```python
from build123d import *

# Parameters (mm, degrees)
F0_W      = 28
F0_H      = 26
F0_R      = 1.55
F1_DEPTH  = 6
F5_DEPTH  = 6.5
F6_DEPTH  = 10
F9_R      = 1.6
F10_DEPTH = 4
F11_DEPTH = 25
F12_START = -6
F9_R_2    = 3.5
F12_DEPTH = 19
F13_R     = 1.6
F14_DEPTH = 4
F15_DEPTH = 25
F16_START = -6
F13_R_2   = 3.5
F16_DEPTH = 19
F17_R     = 3.5
F18_DEPTH = 2
F19_DEPTH = 25


# Not quite as in the source:
# - a fillet or chamfer that OpenCascade refuses, or shapes differently, is made with other operations: its cross-section is extruded or revolved along the edge and cut away or added


with BuildPart() as f1:
    # F0 (on Top) → F1 (new body)
    with BuildSketch(Plane.XY):
        Rectangle(F0_W, F0_H)
        with Locations((0, -7)):
            Circle(F0_R, mode=Mode.SUBTRACT)
        with Locations((-9, 8)):
            Circle(F0_R, mode=Mode.SUBTRACT)
        with Locations((9, 8)):
            Circle(F0_R, mode=Mode.SUBTRACT)
    extrude(amount=F1_DEPTH)

    # F4 (on face) → F5 (join)
    with BuildSketch(Plane(origin=(3.5, 0, -6.0621778265), x_dir=(0.8660254038, 0, 0.5), z_dir=(-0.5, 0, 0.8660254038))):
        with BuildLine():
            Line((12.124355653, -13), (27.124355653, -13))
            ThreePointArc((27.124355653, -13), (14.124355653, 0), (27.124355653, 13))
            Line((27.124355653, 13), (12.124355653, 13))
            Line((12.124355653, 13), (12.124355653, -13))
        make_face()
        with BuildLine():
            ThreePointArc((27.124355653, 13), (14.124355653, 0), (27.124355653, -13))
            ThreePointArc((27.124355653, -13), (36.3167438084, -9.1923881554), (40.124355653, 0))
            ThreePointArc((40.124355653, 0), (36.3167438084, 9.1923881554), (27.124355653, 13))
        make_face()
    extrude(amount=F5_DEPTH)

    # F4 (on face) → F6 (join)
    with BuildSketch(Plane(origin=(3.5, 0, -6.0621778265), x_dir=(0.8660254038, 0, 0.5), z_dir=(-0.5, 0, 0.8660254038))):
        with BuildLine():
            ThreePointArc((27.124355653, 13), (14.124355653, 0), (27.124355653, -13))
            ThreePointArc((27.124355653, -13), (36.3167438084, -9.1923881554), (40.124355653, 0))
            ThreePointArc((40.124355653, 0), (36.3167438084, 9.1923881554), (27.124355653, 13))
        make_face()
    extrude(amount=F6_DEPTH)

    # F7: chamfer of 2 on 1 edges, made by hand

    # F7_s1 → F7_t2 (revolve, cut)
    with BuildSketch(Plane.XZ):
        with BuildLine():
            Line((34.3259853721, 20.9074977067), (31.4393864323, 21.6809595615))
            Line((31.4393864323, 21.6809595615), (31.4193864323, 21.7156005776))
            ThreePointArc((31.4193864323, 21.7156005776), (32.3381910048, 22.1807529184), (33.228711306, 22.694895054))
            Line((33.228711306, 22.694895054), (33.2833523221, 22.6802540378))
            ThreePointArc((33.2833523221, 22.6802540378), (33.7974944577, 21.7897337366), (34.3606263882, 20.9274977067))
            Line((34.3606263882, 20.9274977067), (34.3259853721, 20.9074977067))
        make_face()
    revolve(axis=Axis((21.9903810568, 0, 16.1602540378), (0.5, 0, -0.8660254038)), mode=Mode.SUBTRACT)

    # F8: F1 across plane


with BuildPart() as f1_1:
    add(f1.part)
    add(f1.part.mirror(Plane.YZ))

    # F9 (on face) → F10 (cut)
    with BuildSketch(Plane(origin=(-1.5, 0, 2.5980762114), x_dir=(0.8660254038, 0, 0.5), z_dir=(-0.5, 0, 0.8660254038))):
        with BuildLine():
            ThreePointArc((23.9821806278, -10.5416666667), (27.124355653, -11.0000000001), (30.2665306781, -10.5416666667))
            ThreePointArc((30.2665306781, -10.5416666667), (30.5337260192, -9.7913240209), (30.624355653, -9))
            ThreePointArc((30.624355653, -9), (26.3330316321, -5.5906296338), (23.9821806278, -10.5416666667))
        make_face()
        with Locations((27.124355653, -9)):
            Circle(F9_R, mode=Mode.SUBTRACT)
        with BuildLine():
            ThreePointArc((23.9821806278, -10.5416666667), (27.124355653, -12.5), (30.2665306781, -10.5416666667))
            ThreePointArc((30.2665306781, -10.5416666667), (27.124355653, -11.0000000001), (23.9821806278, -10.5416666667))
        make_face()
        with BuildLine():
            ThreePointArc((22.624355653, 0), (20.2336206122, 3.3195679312), (16.3274806529, 2.1041602206))
            ThreePointArc((16.3274806529, 2.1041602206), (16.1243556529, 0), (16.3274806529, -2.1041602206))
            ThreePointArc((16.3274806529, -2.1041602206), (20.2336206122, -3.3195679312), (22.624355653, 0))
        make_face()
        with Locations((19.124355653, 0)):
            Circle(F9_R, mode=Mode.SUBTRACT)
        with BuildLine():
            ThreePointArc((16.3274806529, -2.1041602206), (16.1243556529, 0), (16.3274806529, 2.1041602206))
            ThreePointArc((16.3274806529, 2.1041602206), (15.624355653, 0), (16.3274806529, -2.1041602206))
        make_face()
        with BuildLine():
            ThreePointArc((30.624355653, 9), (30.5337260192, 9.7913240209), (30.2665306781, 10.5416666667))
            ThreePointArc((30.2665306781, 10.5416666667), (27.124355653, 11.0000000001), (23.9821806278, 10.5416666667))
            ThreePointArc((23.9821806278, 10.5416666667), (26.3330316321, 5.5906296338), (30.624355653, 9))
        make_face()
        with Locations((27.124355653, 9)):
            Circle(F9_R, mode=Mode.SUBTRACT)
        with BuildLine():
            ThreePointArc((23.9821806278, 10.5416666667), (27.124355653, 11.0000000001), (30.2665306781, 10.5416666667))
            ThreePointArc((30.2665306781, 10.5416666667), (27.124355653, 12.5), (23.9821806278, 10.5416666667))
        make_face()
        with BuildLine():
            ThreePointArc((38.124355653, 0), (38.0734566435, 1.0569709078), (37.9212306531, 2.1041602206))
            ThreePointArc((37.9212306531, 2.1041602206), (31.624355653, 0), (37.9212306531, -2.1041602206))
            ThreePointArc((37.9212306531, -2.1041602206), (38.0734566435, -1.0569709078), (38.124355653, 0))
        make_face()
        with Locations((35.124355653, 0)):
            Circle(F9_R, mode=Mode.SUBTRACT)
        with BuildLine():
            ThreePointArc((37.9212306531, -2.1041602206), (38.4439235842, -1.1092649593), (38.624355653, 0))
            ThreePointArc((38.624355653, 0), (38.4439235842, 1.1092649593), (37.9212306531, 2.1041602206))
            ThreePointArc((37.9212306531, 2.1041602206), (38.0734566435, 1.0569709078), (38.124355653, 0))
            ThreePointArc((38.124355653, 0), (38.0734566435, -1.0569709078), (37.9212306531, -2.1041602206))
        make_face()
        with Locations((35.124355653, 0)):
            Circle(F9_R)
        with Locations((19.124355653, 0)):
            Circle(F9_R)
        with Locations((27.124355653, 9)):
            Circle(F9_R)
        with Locations((27.124355653, -9)):
            Circle(F9_R)
    extrude(amount=-F10_DEPTH, mode=Mode.SUBTRACT)

    # F9 (on face) → F11 (cut)
    with BuildSketch(Plane(origin=(-1.5, 0, 2.5980762114), x_dir=(0.8660254038, 0, 0.5), z_dir=(-0.5, 0, 0.8660254038))):
        with Locations((35.124355653, 0)):
            Circle(F9_R)
        with Locations((19.124355653, 0)):
            Circle(F9_R)
        with Locations((27.124355653, -9)):
            Circle(F9_R)
        with Locations((27.124355653, 9)):
            Circle(F9_R)
    extrude(amount=-F11_DEPTH, mode=Mode.SUBTRACT)

    # F9 (on face) → F12 (cut)
    with BuildSketch(Plane(origin=(-1.5, 0, 2.5980762114), x_dir=(0.8660254038, 0, 0.5), z_dir=(-0.5, 0, 0.8660254038)).offset(F12_START)):
        with Locations((27.124355653, 0)):
            Circle(F9_R_2)
    extrude(amount=-F12_DEPTH, mode=Mode.SUBTRACT)

    # F13 (on face) → F14 (cut)
    with BuildSketch(Plane(origin=(1.5, 0, 2.5980762114), x_dir=(0.8660254038, 0, -0.5), z_dir=(0.5, 0, 0.8660254038))):
        with BuildLine():
            ThreePointArc((-25.0201954324, -10.7968750001), (-23.9926978834, -9.56292022), (-23.624355653, -8))
            ThreePointArc((-23.624355653, -8), (-28.687275873, -4.8683422304), (-29.2285158736, -10.7968750001))
            ThreePointArc((-29.2285158736, -10.7968750001), (-27.124355653, -11.0000000001), (-25.0201954324, -10.7968750001))
        make_face()
        with Locations((-27.124355653, -8)):
            Circle(F13_R, mode=Mode.SUBTRACT)
        with BuildLine():
            ThreePointArc((-25.0201954324, 10.7968750001), (-27.124355653, 11.0000000001), (-29.2285158736, 10.7968750001))
            ThreePointArc((-29.2285158736, 10.7968750001), (-28.687275873, 4.8683422304), (-23.624355653, 8))
            ThreePointArc((-23.624355653, 8), (-23.9926978834, 9.56292022), (-25.0201954324, 10.7968750001))
        make_face()
        with Locations((-27.124355653, 8)):
            Circle(F13_R, mode=Mode.SUBTRACT)
        with BuildLine():
            ThreePointArc((-37.6660223197, 3.1421750251), (-38.124355653, 0), (-37.6660223197, -3.1421750251))
            ThreePointArc((-37.6660223197, -3.1421750251), (-34.2731173287, -2.9703394868), (-32.624355653, 0))
            ThreePointArc((-32.624355653, 0), (-34.2731173287, 2.9703394868), (-37.6660223197, 3.1421750251))
        make_face()
        with Locations((-36.124355653, 0)):
            Circle(F13_R, mode=Mode.SUBTRACT)
        with BuildLine():
            ThreePointArc((-16.5826889862, 3.1421750251), (-21.624355653, 0), (-16.5826889862, -3.1421750251))
            ThreePointArc((-16.5826889862, -3.1421750251), (-16.2395420731, -1.5877132403), (-16.1243556529, 0))
            ThreePointArc((-16.1243556529, 0), (-16.2395420731, 1.5877132403), (-16.5826889862, 3.1421750251))
        make_face()
        with Locations((-18.124355653, 0)):
            Circle(F13_R, mode=Mode.SUBTRACT)
        with Locations((-36.124355653, 0)):
            Circle(F13_R)
        with Locations((-18.124355653, 0)):
            Circle(F13_R)
        with Locations((-27.124355653, -8)):
            Circle(F13_R)
        with Locations((-27.124355653, 8)):
            Circle(F13_R)
        with BuildLine():
            ThreePointArc((-37.6660223197, 3.1421750251), (-39.624355653, 0), (-37.6660223197, -3.1421750251))
            ThreePointArc((-37.6660223197, -3.1421750251), (-38.124355653, 0), (-37.6660223197, 3.1421750251))
        make_face()
        with BuildLine():
            ThreePointArc((-16.1243556529, 0), (-16.2395420731, -1.5877132403), (-16.5826889862, -3.1421750251))
            ThreePointArc((-16.5826889862, -3.1421750251), (-15.1540161662, -1.8512383243), (-14.624355653, 0))
            ThreePointArc((-14.624355653, 0), (-15.1540161662, 1.8512383243), (-16.5826889862, 3.1421750251))
            ThreePointArc((-16.5826889862, 3.1421750251), (-16.2395420731, 1.5877132403), (-16.1243556529, 0))
        make_face()
        with BuildLine():
            ThreePointArc((-25.0201954324, -10.7968750001), (-27.124355653, -11.0000000001), (-29.2285158736, -10.7968750001))
            ThreePointArc((-29.2285158736, -10.7968750001), (-27.124355653, -11.5), (-25.0201954324, -10.7968750001))
        make_face()
        with BuildLine():
            ThreePointArc((-25.0201954324, 10.7968750001), (-27.124355653, 11.5), (-29.2285158736, 10.7968750001))
            ThreePointArc((-29.2285158736, 10.7968750001), (-27.124355653, 11.0000000001), (-25.0201954324, 10.7968750001))
        make_face()
    extrude(amount=-F14_DEPTH, mode=Mode.SUBTRACT)

    # F13 (on face) → F15 (cut)
    with BuildSketch(Plane(origin=(1.5, 0, 2.5980762114), x_dir=(0.8660254038, 0, -0.5), z_dir=(0.5, 0, 0.8660254038))):
        with Locations((-18.124355653, 0)):
            Circle(F13_R)
        with Locations((-27.124355653, -8)):
            Circle(F13_R)
        with Locations((-36.124355653, 0)):
            Circle(F13_R)
        with Locations((-27.124355653, 8)):
            Circle(F13_R)
    extrude(amount=-F15_DEPTH, mode=Mode.SUBTRACT)

    # F13 (on face) → F16 (cut)
    with BuildSketch(Plane(origin=(1.5, 0, 2.5980762114), x_dir=(0.8660254038, 0, -0.5), z_dir=(0.5, 0, 0.8660254038)).offset(F16_START)):
        with Locations((-27.124355653, 0)):
            Circle(F13_R_2)
    extrude(amount=-F16_DEPTH, mode=Mode.SUBTRACT)

    # F17 (on face) → F18 (cut)
    with BuildSketch(Plane.XY.offset(6)):
        with Locations((-9, 8)):
            Circle(F17_R)
        with Locations((9, 8)):
            Circle(F17_R)
        with Locations((0, -7)):
            Circle(F17_R)
    extrude(amount=-F18_DEPTH, mode=Mode.SUBTRACT)

    # F17 (on face) → F19 (cut)
    with BuildSketch(Plane.XY.offset(6)):
        with Locations((-9, 8)):
            Circle(F17_R)
        with Locations((9, 8)):
            Circle(F17_R)
        with Locations((0, -7)):
            Circle(F17_R)
    extrude(amount=F19_DEPTH, mode=Mode.SUBTRACT)


solid = f1_1.part
```
CAD build for the part. Positions are in the model's coordinates, mm. A direction names the side the tool comes from. Round coordinates to 2 decimals unless told otherwise and drop trailing zeros. Write each loop counter-clockwise with the first axis right and the second up, starting at its lowest first coordinate (ties: lowest second). Pieces come first, ordered by that corner, then holes.
Item 1: Band-saw the part on A-A on x = 0. Write the cut outline in (y, z).
Filled in:
outline: (-13, 0) - (-8.55, 0) - (-8.55, 4) - (-10.5, 4) - (-10.5, 6) - (-13, 6) - close; (-5.45, 0) - (13, 0) - (13, 6) - (-3.5, 6) - (-3.5, 4) - (-5.45, 4) - close
Item 2: Drop flat-ended pins along their axis: pin 1 Ø2 at (x, y) = (10, 8) entering from +Z; pin 2 Ø5 at (y, z) = (3, 11) entering from -X; pin 3 Ø5 at (y, z) = (-7.5, 15.5) entering from -X. Give the stop position or say it passes through.
Filled in:
pin 1: stops at z = 4
pin 2: stops at x = -37.38
pin 3: stops at x = -36.87
Item 3: Tool access for faces 1 (the flat face through (10, 6, 4)), 2 (the cylindrical face through (-8.285, 6.625, 1.972)), 3 (the flat face through (12.05, 0.06, 6.38)), 4 (the flat face through (21.859, 0.148, 16.085)), 5 (the flat face through (23.26, 0.182, 5.346)): list every direction of +Z, -Z, +X, -X, +Y, -Y with a clear straight run to the whole face (end or side of a thin tool).
Filled in:
face 1: +Z
face 2: +Z, -Z
face 3: none
face 4: +Z, +Y, -Y
face 5: -Z, +X, +Y, -Y
Item 4: Band-saw the part on B-B on z = 5. Give the number of separate pieces and of enclosed holes in the cut face, then the cut area to 3 significant figures.
Filled in:
separate pieces: 1
enclosed holes: 5
area: 1,040 mm2
Item 5: Mould opens along Y. For faces 6 (the flat face through (0, -13, 5)), 7 (the flat face through (-12.05, 0.06, 6.38)), 8 (the cylindrical face through (9.715, 6.625, 1.972)) say: released by +Y, released by -Y, zero draft, split by the parting line, or undercut.
Filled in:
face 6: released by -Y
face 7: zero draft
face 8: undercut
Item 6: Drill centre lines: L1, parallel to X at y = 8, z = 4.6; L2, parallel to Y at x = 0, z = 4.5; L3, parallel to Y at x = 25.5, z = 13. Where is each one in solid material? Low to high.
Filled in:
L1: x = -21.97 to -12.5, -5.5 to 5.5, 12.5 to 21.97
L2: y = -13 to -10.5, -3.5 to 13
L3: y = -12.92 to -9.66, -8.34 to 8.34, 9.66 to 12.92
